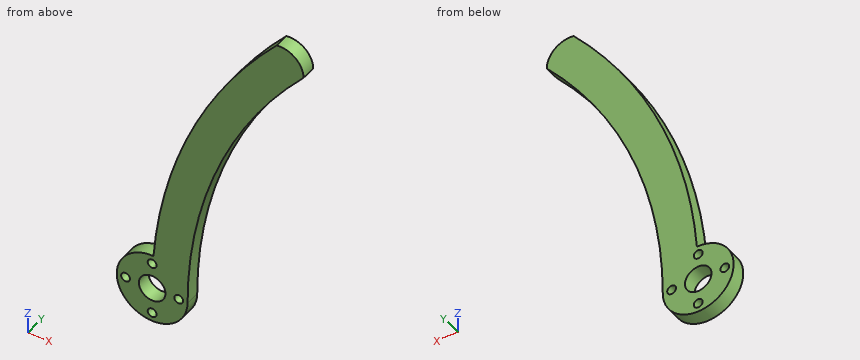
from build123d import *

# Parameters (mm, degrees)
ESQUISSE1_R             = 4.5
BOSS_EXTRU_1_DEPTH      = 5
ESQUISSE2_R             = 1.5
ENL_V_MAT_EXTRU_1_DEPTH = 5


with BuildPart() as part:
    # Esquisse1 → Boss.-Extru.1 (new body)
    with BuildSketch(Plane(origin=(0, 0, 0), x_dir=(1, 0, 0), z_dir=(0, 1, 0))):
        with BuildLine():
            ThreePointArc((-148, 0), (-168.642916175, 8.324662155), (-159.55, -11.991559532))
            ThreePointArc((-159.55, -11.991559532), (-146.800083184, -63.637532772), (-117.822638991, -108.24890642))
            ThreePointArc((-117.822638991, -108.24890642), (-111.47655915, -106.418874078), (-108.723180083, -100.415487414))
            ThreePointArc((-108.723180083, -100.415487414), (-137.831474367, -53.911823136), (-148, 0))
        make_face()
        with Locations((-160, 0)):
            Circle(ESQUISSE1_R, mode=Mode.SUBTRACT)
    extrude(amount=BOSS_EXTRU_1_DEPTH)

    # Esquisse2 → Enlèv. mat.-Extru.1 (cut)
    with BuildSketch(Plane(origin=(0, 5, 0), x_dir=(1, 0, 0), z_dir=(0, 1, 0))):
        with Locations((-151, 0)):
            Circle(ESQUISSE2_R)
        with Locations((-160, -9)):
            Circle(ESQUISSE2_R)
        with Locations((-169, 0)):
            Circle(ESQUISSE2_R)
        with Locations((-160, 9)):
            Circle(ESQUISSE2_R)
    extrude(amount=-ENL_V_MAT_EXTRU_1_DEPTH, mode=Mode.SUBTRACT)


solid = part.part
Geometry: final body of the model. Coordinates: model frame, mm. Round coordinates to 2 decimals unless told otherwise and drop trailing zeros. Loops run counter-clockwise (first coordinate to the right, second up) from the corner with the lowest first, then second, coordinate; pieces in that order, holes last. Notation, with made-up numbers: M 30.5,-17.75 L 37.5,-17.75 A21 ccw 37.5,0.25 Z; hole C 80.25,53.5 d8. An arc over 180 degrees is marked long. Put each result on its own line as item: value. Start each with the question number.
(1) Material intervals for line 1 along Z through (x, y) = (-160, 1.2); line 2 along X through (y, z) = (2.4, -9); line 3 along X through (y, z) = (3, -3.5), sorted ascending. Write a range as [from, to].
(2) Section query A-A (y = 0.8). Return loops of the section in (x, z), then the cut area to 3 significant figures.
(3) Section query C-C (z = 17). Return loops of the section in (x, y), then the cut area to 3 significant figures.
(4) Contact query for flat-ended pins moving along their axis: pin 1 Ø5.5 at (x, z) = (-160, 0) entering from -Y; pin 2 Ø3 at (x, y) = (-119.5, 2.5) entering from -Z; pin 3 Ø2 at (y, z) = (4, 69.5) entering from -X. Output: stop coordinate, or through.
(5) Section query D-D (x = -133). Return loops of the section in (y, z), then the cut area to 3 significant figures.
(6) Section query B-B (x = -151). Return loops of the section in (y, z).
Findings below:
1. line 1: z = [-12, -10.5], [-7.5, -4.5], [4.5, 7.5], [10.5, 12]
1. line 2: x = [-167.94, -161.5], [-158.5, -152.06]
1. line 3: x = [-171.48, -162.83], [-157.17, -148.52]
2. outline: M -159.55,11.99 A12 ccw long -148,0 A148 cw -108.72,100.42 A7.92 ccw -117.82,108.25 A160 ccw Z; hole C -169,0 d3; hole C -160,0 d9; hole C -160,-9 d3; hole C -160,9 d3; hole C -151,0 d3
2. area: 1,650 mm2
3. outline: M -159.09,0 L -147.02,0 L -147.02,5 L -159.09,5 Z
3. area: 60.4 mm2
4. pin 1: passes through
4. pin 2: stops at z = 85.22
4. pin 3: stops at x = -144.6
5. outline: M 0,64.92 L 5,64.92 L 5,88.94 L 0,88.94 Z
5. area: 120 mm2
6. outline: M 0,-7.94 L 5,-7.94 L 5,-1.5 L 0,-1.5 Z; M 0,1.5 L 5,1.5 L 5,52.91 L 0,52.91 Z
